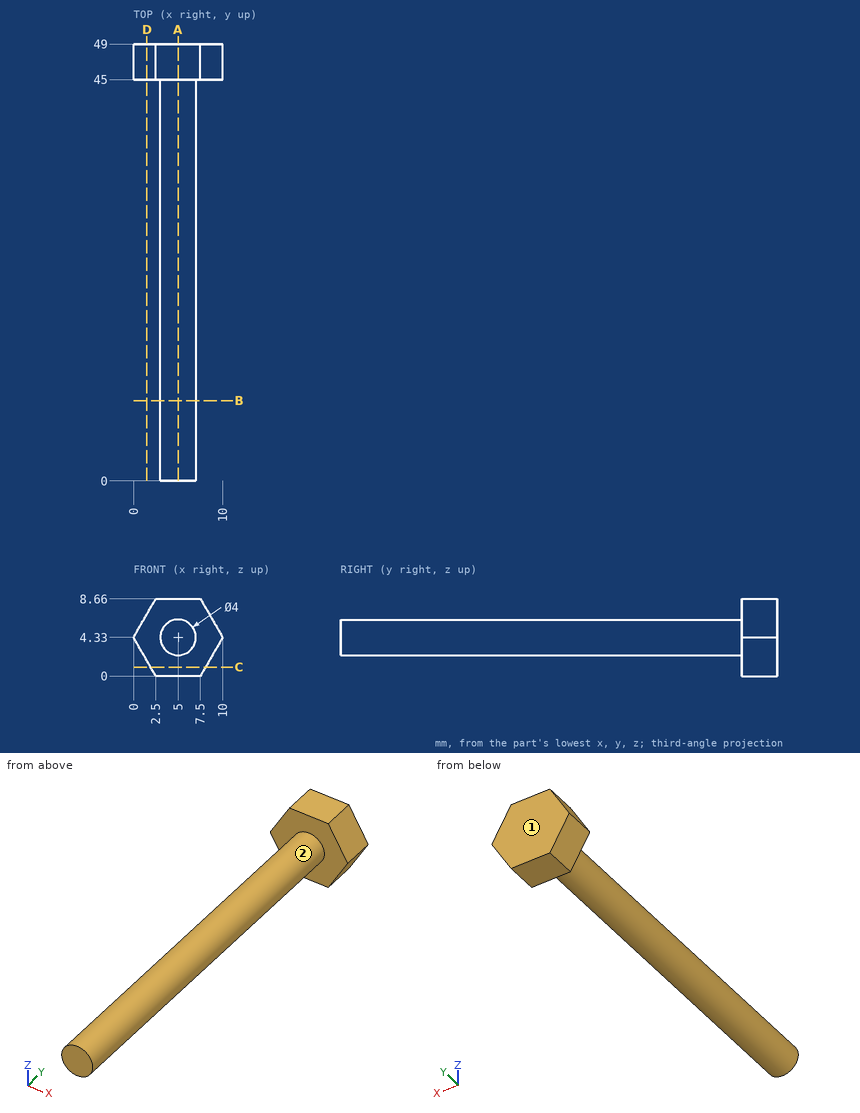
Part print with two shaded views. Sizes in mm from the minimum x, y, z corner. A direction names the side the tool comes from. Coordinates: 2 decimals unless noted, no trailing zeros. Order: outer loops, then holes, each group sorted by start corner. A loop starts at its lowest first (then second) coordinate and runs counter-clockwise, first axis right, second up. Notation, with made-up numbers: M 35.5,-39 L 80.5,-39 A10 cw 80.5,-33 Z; hole C -31.5,88 d6. An arc over 180 degrees is marked long. One line per question, with ' | ' between items. Start each with the question number.
1. Flat gauge pins, fed straight in: P1, Ø2, axis at x = 6.5, z = 6, coming from the -Y side; P2, Ø5, axis at x = 2.5, y = 30.5, coming from the +Z side; P3, Ø2, axis at y = 41.5, z = 3, coming from the +X side. Where does each tip first touch, or does it go through?
2. Cut at D-D (x = 1.5). Write the cut outline in (y, z), plus the area to 3 significant figures.
3. Cut at B-B (y = 9). Write the cut outline in (x, z), plus the area to 3 significant figures.
4. Tool access for the marked faces 1 and 2: list every direction of +Z, -Z, +X, -X, +Y, -Y with a clear straight run to the whole face (end or side of a thin tool).
5. Wall check: line 1 along Y through (x, z) = (5.25, 1.5); line 2 along X through (y, z) = (16.5, 4.5); line 3 along X through (y, z) = (44, 5.75). Give the ranges that are in metal, low to high. Write a range as [from, to].
6. Cut at C-C (z = 1). Write the cut outline in (x, y).
7. Cut at A-A (x = 5). Write the cut outline in (y, z), plus the area to 3 significant figures.
The answers:
1) P1: stops at y = 0 | P2: stops at z = 6.33 | P3: stops at x = 6.97
2) outline: M 45,1.73 L 49,1.73 L 49,6.93 L 45,6.93 Z | area: 20.8 mm2
3) outline: C 5,4.33 d4 | area: 12.6 mm2
4) face 1: +Z, -Z, +X, -X, +Y | face 2: -Y
5) line 1: y = [45, 49] | line 2: x = [3.01, 6.99] | line 3: x = [3.59, 6.41]
6) outline: M 1.92,45 L 8.08,45 L 8.08,49 L 1.92,49 Z
7) outline: M 0,2.33 L 45,2.33 L 45,0 L 49,0 L 49,8.66 L 45,8.66 L 45,6.33 L 0,6.33 Z | area: 215 mm2
